Geometry: final body of the model. Coordinates: model frame, mm. Face numbers are marked on the shaded views. A direction names the side the tool comes from. Coordinates: 2 decimals unless noted, no trailing zeros. Order: outer loops, then holes, each group sorted by start corner. A loop starts at its lowest first (then second) coordinate and runs counter-clockwise, first axis right, second up. Notation, with made-up numbers: M 81.25,47 L 127.25,47 A30 cw 127.25,72 Z; hole C 35.5,4.25 d6. An arc over 180 degrees is marked long. Write item = value, one per line.
Autodesk Inventor part; units mm, degrees
ref_plane "Work Plane2" through (-10, -10, -4.4) normal (0, 0, 1) x (1, 0, 0)
ref_plane "YZ Plane" through (0, 0, 0) normal (1, 0, 0) x (0, 1, 0)
ref_plane "XZ Plane" through (0, 0, 0) normal (0, 1, 0) x (-1, 0, 0)
ref_plane "Work Plane1" through (0, 0, -6.6) normal (0, 0, -1) x (-1, 0, 0)
sketch "Sketch1" plane through (0, 0, -6.6) normal (0, 0, -1) x (-1, 0, 0)
  circle A0 centre (3.0857, 5.1173) radius 10
  line L0 (-6.9143, 5.1173) -> (-6.9143, 18.1173)
  line L1 (-6.9143, 18.1173) -> (13.0857, 18.1173)
  line L2 (13.0857, 18.1173) -> (13.0857, 5.1173)
  circle A1 centre (0, 0) radius 5
  point P0 (0, 0)
  dimension "d24" = 13
  dimension "d25" = 20
ref_plane "Work Plane2" through (-10, -10, -4.4) normal (0, 0, 1) x (1, 0, 0)
extrude "Extrusion1" add sketch "Sketch1" along normal blind 2 contours A0 A1 | A0 L0 L1 L2 | A0 A1 picked at (6.1055, 10.6249) picked at (0.8611, -2.5748)
sketch "Sketch9" plane through (0, 0, -8.6) normal (0, 0, -1) x (-1, 0, 0)
  circle A0 centre (3.0857, 5.1173) radius 5 construction
  arc A1 (-6.9143, 5.1173) -> (13.0857, 5.1173) centre (3.0857, 5.1173) ccw
  circle A2 centre (3.0857, 5.1173) radius 3.75
  dimension "d43" = 7.5
extrude "Extrusion6" cut sketch "Sketch9" against normal up to surface (2 mm away)
sketch "Sketch10" plane through (0, 0, -8.6) normal (0, 0, -1) x (-1, 0, 0)
  arc A0 (-6.9143, 5.1173) -> (13.0857, 5.1173) centre (3.0857, 5.1173) ccw
  line L0 (3.0857, -4.8827) -> (3.0857, -2.8827)
  line L1 (3.0857, -2.8827) -> (4.5857, -2.8827)
  line L2 (4.5857, -2.8827) -> (3.0857, -2.8827)
  line L3 (-2.1325, -2.8827) -> (-2.1325, -5.7607)
  line L4 (4.5857, -2.8827) -> (4.5857, -3.3119)
  line L5 (-2.1325, -5.7607) -> (-2.1325, -7.2943)
  line L6 (4.5857, -3.3119) -> (4.5857, -2.7408)
  line L7 (-4, 15) -> (-4, 13) construction
  line L8 (4, 13) -> (4, 15) construction
  line L9 (13.0857, 18.1173) -> (-6.9143, 18.1173)
  line L10 (-6.9143, 18.1173) -> (13.0857, 18.1173)
  line L11 (-6.9143, 18.1173) -> (-6.9143, 5.1173)
  line L12 (13.0857, 18.1173) -> (13.0857, 5.1173)
  arc A1 (-6.9143, 5.1173) -> (13.0857, 5.1173) centre (3.0857, 5.1173) ccw
  circle A2 centre (3.0857, 5.1173) radius 6.5
  line L13 (3.0857, 5.1173) -> (3.0857, 11.6173) construction
  line L14 (3.0857, 11.6173) -> (7.0857, 11.6173)
  line L15 (7.0857, 11.6173) -> (3.0857, 11.6173)
  line L16 (3.0857, 11.6173) -> (-0.9143, 11.6173)
  line L17 (-0.9143, 10.2408) -> (-0.9143, 18.1173)
  line L18 (-0.9143, 18.1173) -> (7.0857, 18.1173)
  line L19 (7.0857, 18.1173) -> (7.0857, 10.2408)
  point P0 (5.6921, -0.9362)
  dimension "d31" = 2
  dimension "d37" = 1.5
  dimension "d44" = 4
  dimension "d45" = 4
extrude "Extrusion8" cut sketch "Sketch10" against normal up to next contours A0 L11 L9 L17 A2 L19 L12
sketch "Sketch11" plane through (0, 0, -8.6) normal (0, 0, -1) x (-1, 0, 0)
  line L0 (7.0857, 18.1173) -> (-0.9143, 18.1173)
  line L1 (7.0857, 18.1173) -> (7.0857, 21.6173)
  line L2 (7.0857, 21.6173) -> (-0.9143, 21.6173)
  line L3 (-0.9143, 21.6173) -> (-0.9143, 18.1173)
  point P0 (0, 0)
  dimension "d46" = 3.5
extrude "Extrusion9" add sketch "Sketch11" against normal up to surface (2 mm away)
sketch "Sketch13" plane through (0, 0, -6.6) normal (0, 0, 1) x (1, 0, 0)
  circle A0 centre (-3.0857, 5.1173) radius 3.75
  arc A1 (6.0076, 10.3673) -> (-3.0857, 15.6173) centre (-3.0857, 5.1173) ccw
  line L0 (-3.0857, 5.1173) -> (6.0076, 10.3673) construction
  arc A2 (-3.0857, 15.6173) -> (-12.1789, 10.3673) centre (-3.0857, 5.1173) ccw
  line L1 (-3.0857, 5.1173) -> (-12.1789, 10.3673) construction
  arc A3 (6.0076, 10.3673) -> (-12.1789, 10.3673) centre (-3.0857, 5.1173) ccw
  arc A4 (6.8736, 10.8673) -> (-13.045, 10.8673) centre (-3.0857, 5.1173) ccw
  line L2 (-12.1789, 10.3673) -> (-13.045, 10.8673)
  line L3 (6.0076, 10.3673) -> (6.8736, 10.8673)
  arc A5 (-7.0857, 10.2408) -> (0.9143, 10.2408) centre (-3.0857, 5.1173) ccw
  line L4 (-3.0857, 5.1173) -> (-3.0857, 15.6173)
  point P0 (0, 0)
  point P1 (-3.0857, 16.6173)
  dimension "d60" = 120
  dimension "d61" = 11.5
  dimension "d65" = 10.5
  dimension "d66" = 1
extrude "Extrusion11" add sketch "Sketch13" along normal blind 10 contours A2 L2 A4 L3 A1
equation "\"d60\" = 2 * d56"
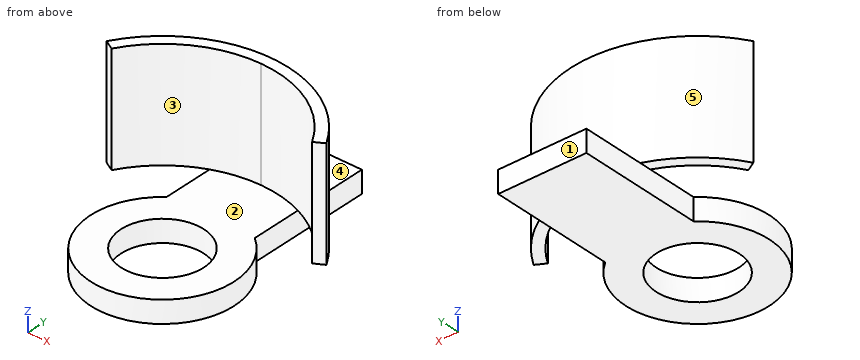
1) Set-up query: the marked faces 1 and 2. Return all of +Z, -Z, +X, -X, +Y, -Y with unobstructed straight access to the full face (end or side cutting, diameter ignored); none if empty.
Numbers:
face_1 = +Z, -Z, +X, -X, +Y
face_2 = +Z, -Y
2) Line query: L1, parallel to X at y = 12, z = 1.25; L2, parallel to X at y = 13.5, z = -7.5; L3, parallel to Z at x = -5, y = 18.25. Output: solid intervals per line, ascending.
Numbers:
L1 = -12.3 to -11.02, 4.84 to 6.13
L2 = -7.09 to 0.91
L3 = -8.6 to -6.6
3) Section D-D, the plane x = -2.5. Return loops of the section in (y, z).
Numbers:
outline = M -1.36,-8.6 L 1.41,-8.6 L 1.41,-6.6 L -1.36,-6.6 Z; M 8.82,-8.6 L 21.62,-8.6 L 21.62,-6.6 L 16.6,-6.6 L 16.6,3.4 L 15.6,3.4 L 15.6,-6.6 L 8.82,-6.6 Z
4) Section C-C, the plane z = 0.25. Return loops of the section in (x, y) (3 decimals).
Numbers:
outline = M -13.045,10.867 L -12.179,10.367 A10.5 cw -3.086,15.617 A10.5 cw 6.008,10.367 L 6.874,10.867 A11.5 ccw Z
5) Pin query (flat end, axial travel): pin 1 (4 mm diameter, centred on y = 6.5, z = -6, fed in from -X); pin 2 (3 mm diameter, centred on x = -10.5, y = 13, fed in from -Z); pin 3 (8 mm diameter, centred on x = -9.5, y = 3, fed in from +Z); pin 4 (10 mm diameter, centred on x = -3.09, y = 5.12, fed in from -Z). Return the tip coordinate at first contact, or that it passes through.
Numbers:
pin_1 = -9.59
pin_2 = -6.6
pin_3 = -6.6
pin_4 = -8.6
6) Mould query, pull axis X, two halves, no side actions, for the marked faces 3, 4 and 5. Classes: pulls with the +X half, pulls with the -X half, needs draft (parallel to the pull), parting line crosses it, or undercut.
Numbers:
face_3 = undercut
face_4 = needs draft
face_5 = parting line crosses it
7) Section B-B, the plane y = 2. Return loops of the section in (x, z).
Numbers:
outline = M -8.79,-8.6 L -5.17,-8.6 L -5.17,-6.6 L -8.79,-6.6 Z; M -1,-8.6 L 2.62,-8.6 L 2.62,-6.6 L -1,-6.6 Z
8) Section A-A, the plane x = -8.75. Return loops of the section in (y, z).
Numbers:
outline = M 1.93,-8.6 L 8.31,-8.6 L 8.31,-6.6 L 1.93,-6.6 Z; M 13.96,-6.6 L 15.13,-6.6 L 15.13,3.4 L 13.96,3.4 Z
